from build123d import *

# Parameters (mm, degrees)
SKETCH1_R             = 11
BOSS_EXTRUDE1_DEPTH   = 2
SKETCH2_R             = 5
BOSS_EXTRUDE2_DEPTH   = 10
CUT_EXTRUDE1_REACH    = 21.647
SKETCH3_R             = 3
SKETCH5_W             = 1.25
SKETCH5_H             = 5
F_3_0MM_DOWEL_HOLE1_D = 3


with BuildPart() as part:
    # Sketch1 → Boss-Extrude1 (new body)
    with BuildSketch(Plane.XY):
        Circle(SKETCH1_R)
    extrude(amount=BOSS_EXTRUDE1_DEPTH)

    # Sketch2 → Boss-Extrude2 (add)
    with BuildSketch(Plane.XY.offset(2)):
        Circle(SKETCH2_R)
    extrude(amount=BOSS_EXTRUDE2_DEPTH)

    # Sketch3 → Cut-Extrude1 (cut, up to next)
    with BuildSketch(Plane.XY.offset(12), mode=Mode.PRIVATE) as cut_extrude1_sk1:
        Circle(SKETCH3_R)
    cut_extrude1_tool1 = extrude(cut_extrude1_sk1.sketch, amount=-CUT_EXTRUDE1_REACH, mode=Mode.PRIVATE) & part.part
    add(cut_extrude1_tool1.solids().sort_by_distance((0, 0, 12))[0], mode=Mode.SUBTRACT)

    # Sketch5 → Tap Drill for M3x0.5 Tap1 (revolve, cut)
    with BuildSketch(Plane(origin=(0, 0, 7), x_dir=(0, 0, -1), z_dir=(1, 0, 0))):
        with Locations((0.625, 2.5)):
            Rectangle(SKETCH5_W, SKETCH5_H)
    revolve(axis=Axis((0, -6.35, 7), (0, 1, 0)), mode=Mode.SUBTRACT)

    # Ø3.0mm Dowel Hole1 (through all)
    with Locations(Plane.XY.offset(2)):
        with Locations((5.656854249, 5.656854249), (-5.656854249, -5.656854249), (-5.656854249, 5.656854249), (5.656854249, -5.656854249)):
            Hole(F_3_0MM_DOWEL_HOLE1_D / 2)


solid = part.part
CAD build for the part. Positions are in the model's coordinates, mm. A direction names the side the tool comes from. Coordinates: 2 decimals unless noted, no trailing zeros. Order: outer loops, then holes, each group sorted by start corner. A loop starts at its lowest first (then second) coordinate and runs counter-clockwise, first axis right, second up.
Item 1: Band-saw the part on A-A on x = 0. List the corners of the cut face in (y, z), plus the area to 3 significant figures.
Check sheet entries:
outline: (-11, 0) - (-3, 0) - (-3, 12) - (-5, 12) - (-5, 2) - (-11, 2) - close; (3, 0) - (11, 0) - (11, 2) - (5, 2) - (5, 5.75) - (3, 5.75) - close; (3, 8.25) - (5, 8.25) - (5, 12) - (3, 12) - close
area: 67.0 mm2
Item 2: Pin check, flat tips, straight feed: pin 1 Ø12 at (x, y) = (1.5, 0.5) entering from -Z; pin 2 Ø4 at (x, y) = (-5.66, 5.66) entering from +Z; pin 3 Ø2 at (x, z) = (0, 7) entering from -Y; pin 4 Ø3 at (y, z) = (7.5, 3) entering from +X. Stop position of each tip, or through.
Check sheet entries:
pin 1: stops at z = 0
pin 2: stops at z = 2
pin 3: stops at y = -5
pin 4: stops at x = 8.96
Item 3: Drill centre lines: L1, parallel to Y at x = 0, z = 8.75; L2, parallel to X at y = 4, z = 7; L3, parallel to X at y = -5.5, z = 0.75. Where is each one in solid material? Low to high.
Check sheet entries:
L1: y = -5 to -3, 3 to 5
L2: x = -3 to -1.25, 1.25 to 3
L3: x = -9.53 to -7.15, -4.17 to 4.17, 7.15 to 9.53
Item 4: 3-axis set-ups, long thin cutter, end or side, ignore diameter. For faces 4 (the face through (-0.05, 3.88, 8.25)), 5 (the face through (2.3, -2.3, 0)), 6 (the face through (2, -5, 2)): which of +Z, -Z, +X, -X, +Y, -Y reach the whole face in a straight line?
Check sheet entries:
face 4: +Y
face 5: -Z, +X, -X, +Y, -Y
face 6: +Z
Item 5: Band-saw the part on D-D on x = 6.25. List the corners of the cut face in (y, z), plus the area to 3 significant figures.
Check sheet entries:
outline: (-9.05, 0) - (-7.03, 0) - (-7.03, 2) - (-9.05, 2) - close; (-4.28, 0) - (4.28, 0) - (4.28, 2) - (-4.28, 2) - close; (7.03, 0) - (9.05, 0) - (9.05, 2) - (7.03, 2) - close
area: 25.2 mm2
Item 6: Band-saw the part on B-B on y = 0. List the corners of the cut face in (x, z), plus the area to 3 significant figures.
Check sheet entries:
outline: (-11, 0) - (-3, 0) - (-3, 12) - (-5, 12) - (-5, 2) - (-11, 2) - close; (3, 0) - (11, 0) - (11, 2) - (5, 2) - (5, 12) - (3, 12) - close
area: 72.0 mm2
Item 7: Band-saw the part on C-C on z = 3. List the corners of the cut face in (x, y).
Check sheet entries:
outline: circle Ø10 at (0, 0); hole circle Ø6 at (0, 0)
Item 8: Two-plate mould, pull along X, no slides. Class faces 1 (the face through (-0.65, -2.93, 6.08)), 2 (the face through (-2.38, -10.74, 0.99)), 3 (the face through (-0.1, -3.3, 12)): +X half, -X half, draft (parallel to the pull), parting line (faces both ways), or undercut.
Check sheet entries:
face 1: undercut
face 2: parting line
face 3: draft
